```python
from build123d import *

# Parameters (mm, degrees)
BOSS_EXTRUDE1_DEPTH     = 4.7625
SKETCH2_R               = 1.905
CUT_EXTRUDE1_DEPTH      = 1
CUT_EXTRUDE1_DEPTH_BACK = 74.025
FILLET1_R               = 9.525


with BuildPart() as part:
    # Sketch1 → Boss-Extrude1 (new body, symmetric)
    with BuildSketch(Plane.XY):
        Polygon((33.3375, -46.0375), (36.5125, -46.0375), (36.5125, 46.0375), (-36.5125, 46.0375), (-36.5125, -46.0375), (-33.3375, -46.0375), (-33.3375, 42.8625), (33.3375, 42.8625), align=None)
    extrude(amount=BOSS_EXTRUDE1_DEPTH, both=True)

    # Sketch2 → Cut-Extrude1 (cut, two sides)
    with BuildSketch(Plane.ZY.offset(36.5125)) as cut_extrude1_sk:
        with Locations((0, -39.6875)):
            Circle(SKETCH2_R)
        with BuildLine():
            Line((-4.7625, -39.6875), (-4.7625, -46.0375))
            Line((-4.7625, -46.0375), (4.7625, -46.0375))
            Line((4.7625, -46.0375), (4.7625, -39.6875))
            ThreePointArc((4.7625, -39.6875), (0, -44.45), (-4.7625, -39.6875))
        make_face()
    extrude(amount=CUT_EXTRUDE1_DEPTH, mode=Mode.SUBTRACT)
    extrude(cut_extrude1_sk.sketch, amount=-CUT_EXTRUDE1_DEPTH_BACK, mode=Mode.SUBTRACT)

    # Fillet1
    fillet1_edges = [part.edges().sort_by_distance(p)[0] for p in [
        (33.3375, 42.8625, 0),
        (-33.3375, 42.8625, 0),
        (-36.5125, 46.0375, 0),
        (36.5125, 46.0375, 0),
    ]]
    fillet(fillet1_edges, radius=FILLET1_R)


solid = part.part
```
Model file for the job. Use its own axes, mm. A direction names the side the tool comes from. Give positions to 0.01 mm unless a question says otherwise; leave off trailing zeros. Write each loop counter-clockwise with the first axis right and the second up, starting at its lowest first coordinate (ties: lowest second). Pieces come first, ordered by that corner, then holes. Notation, with made-up numbers: (-24.75, 37) - (15.25, 37) arc R26 cw to (15.25, 57) - close; hole circle Ø2 at (-16, 31). An arc over 180 degrees is marked (long way). One line per question, with ' | ' between items. Start each with the question number.
(1) Slice it at A-A on y = -21.5. Write the cut outline in (x, z).
(2) 3-axis set-ups, long thin cutter, end or side, ignore diameter. For faces 1 (the face through (36.512, -5, 0)), 2 (the face through (-30.47, 40.15, -0.07)): which of +Z, -Z, +X, -X, +Y, -Y reach the whole face in a straight line?
(3) Two-plate mould, pull along Z, no slides. Class faces 3 (the face through (0, 45, -4.762)), 4 (the face through (0, 42.862, 0)), 5 (the face through (-34.95, -37.8, -0.25)): +Z half, -Z half, draft (parallel to the pull), parting line (faces both ways), or undercut.
(4) Slice it at C-C on x = -22. Write the cut outline in (y, z).
(5) Slice it at D-D on y = 35. Write the cut outline in (x, z), plus the area to 3 significant figures.
(6) Pin check, flat tips, straight feed: P1, Ø4, axis at x = 28.5, z = 1.5, coming from the -Y side; P2, Ø3, axis at x = -11.5, z = 0.5, coming from the -Y side. Stop position of each tip, or through.
(7) Slice it at B-B on z = 0. Give the number of separate pieces and of enclosed holes in the cut face, plus the area to 3 significant figures.
(8) Wall check: line 1 along X through (y, z) = (14, 1.75); line 2 along Y through (x, z) = (15, 2); line 3 along X through (y, z) = (35.5, 4). Give the ranges that are in metal, low to high. Write a range as from..to.
Results below:
1) outline: (-36.51, -4.76) - (-33.34, -4.76) - (-33.34, 4.76) - (-36.51, 4.76) - close; (33.34, -4.76) - (36.51, -4.76) - (36.51, 4.76) - (33.34, 4.76) - close
2) face 1: +Z, -Z, +X, +Y, -Y | face 2: +Z, -Z, -Y
3) face 3: -Z half | face 4: draft | face 5: undercut
4) outline: (42.86, -4.76) - (46.04, -4.76) - (46.04, 4.76) - (42.86, 4.76) - close
5) outline: (-36.51, -4.76) - (-33.19, -4.76) - (-33.19, 4.76) - (-36.51, 4.76) - close; (33.19, -4.76) - (36.51, -4.76) - (36.51, 4.76) - (33.19, 4.76) - close | area: 63.3 mm^2
6) P1: y = 40.12 | P2: y = 42.86
7) separate pieces: 3 | enclosed holes: 0 | area: 762 mm^2
8) line 1: -36.51..-33.34, 33.34..36.51 | line 2: 42.86..46.04 | line 3: -36.51..-33.09, 33.09..36.51
